from build123d import *

# Parameters (mm, degrees)
F1_W     = 65
F1_H     = 60
F1_R     = 2.5
F2_DEPTH = 1.5
F3_W     = 65
F3_H     = 1.5
F4_DEPTH = 25
F5_R     = 2
F6_DEPTH = 25
F7_R     = 2


with BuildPart() as f2:
    # F1 (on face) → F2 (new body)
    with BuildSketch(Plane.XZ):
        with Locations((32.5, -30)):
            Rectangle(F1_W, F1_H)
        with BuildLine():
            ThreePointArc((55, -45), (57.5, -47.5), (55, -50))
            ThreePointArc((55, -50), (34.847457, -41.652543), (26.5, -21.5))
            ThreePointArc((26.5, -21.5), (29, -19), (31.5, -21.5))
            ThreePointArc((31.5, -21.5), (38.382991, -38.117009), (55, -45))
        make_face(mode=Mode.SUBTRACT)
        with Locations((55, -21.5)):
            Circle(F1_R, mode=Mode.SUBTRACT)
    extrude(amount=F2_DEPTH)

    # F3 (on Front) → F4 (join)
    with BuildSketch(Plane.XZ):
        with Locations((32.5, -0.75)):
            Rectangle(F3_W, F3_H)
    extrude(amount=-F4_DEPTH)

    # F5 (on face) → F6 (cut)
    with BuildSketch(Plane.XY):
        with Locations((53, 12.5)):
            Circle(F5_R)
        with Locations((12, 12.5)):
            Circle(F5_R)
    extrude(amount=-F6_DEPTH, mode=Mode.SUBTRACT)

    # F7
    f7_edges = [f2.edges().sort_by_distance(p)[0] for p in [
        (65, -0.75, -60),
        (32.5, 0, -1.5),
        (32.5, -1.5, 0),
        (0, -0.75, -60),
        (0, 25, -0.75),
        (65, 25, -0.75),
    ]]
    fillet(f7_edges, radius=F7_R)


solid = f2.part
Geometry: final body of the model. Coordinates: model frame, mm. A direction names the side the tool comes from. Give positions to 0.01 mm unless a question says otherwise; leave off trailing zeros. Order: outer loops, then holes, each group sorted by start corner. A loop starts at its lowest first (then second) coordinate and runs counter-clockwise, first axis right, second up. Notation, with made-up numbers: (1, -0.5) - (9, -0.5) arc R15 cw to (9, 16.5) - close; hole circle Ø4 at (-15.75, 67). An arc over 180 degrees is marked (long way). Use CSV: the item, a comma, the result in double quotes.
1. Section query B-B (y = 13.5). Output: boundary loops of the cut face in (x, z).
Answers below:
outline,"(0, -1.5) - (10.27, -1.5) - (10.27, 0) - (0, 0) - close; (13.73, -1.5) - (51.27, -1.5) - (51.27, 0) - (13.73, 0) - close; (54.73, -1.5) - (65, -1.5) - (65, 0) - (54.73, 0) - close"
2. Section query C-C (z = -47.5). Output: boundary loops of the cut face in (x, y).
Answers below:
outline,"(0, -1.5) - (43.33, -1.5) - (43.33, 0) - (0, 0) - close; (57.5, -1.5) - (65, -1.5) - (65, 0) - (57.5, 0) - close"
3. Contact query for flat-ended pins moving along their axis: pin 1 (5 mm diameter, centred on x = 14, y = 22, fed in from -Z); pin 2 (3 mm diameter, centred on x = 51.5, y = 2.5, fed in from -Z). Output: stop coordinate, or through.
Answers below:
pin 1,"z = -1.5"
pin 2,"z = -1.77"
4. Mould query, pull axis Z, two halves, no side actions, for faces 1 (the face through (0.57, -0.76, -59.4)), 2 (the face through (35.1, -0.7, -41.9)), 3 (the face through (10.526, 13.852, -0.74)). Classes: +Z half, -Z half, draft (parallel to the pull), parting line (faces both ways), or undercut.
Answers below:
face 1,"-Z half"
face 2,"undercut"
face 3,"draft"
5. Access query for faces 4 (the face through (32, 0, -25)), 5 (the face through (0.57, 24.4, -0.74)), 6 (the face through (38.2, -0.74, -37.93)). Directions: +Z, -Z, +X, -X, +Y, -Y. A direction counts if a zero-diameter tool reaches every point of the face in a straight line with its end or side. Return the directions, or none.
Answers below:
face 4,"-Z, +X, -X, +Y"
face 5,"+Z, -Z, -X, +Y"
face 6,"+Y, -Y"
6. Material intervals for line 1 along Y through (x, z) = (32.5, -24); line 2 along Y through (x, z) = (53, -0.85), sorted ascending. Write a range as from..to.
Answers below:
line 1,"-1.5..0"
line 2,"-1.14..10.5, 14.5..25"
7. Section query A-A (z = -23). Output: boundary loops of the cut face in (x, y).
Answers below:
outline,"(0, -1.5) - (26.54, -1.5) - (26.54, 0) - (0, 0) - close; (31.55, -1.5) - (53, -1.5) - (53, 0) - (31.55, 0) - close; (57, -1.5) - (65, -1.5) - (65, 0) - (57, 0) - close"
8. Section query D-D (y = 6.25). Output: boundary loops of the cut face in (x, z), plus the area to 3 significant figures.
Answers below:
outline,"(0, -1.5) - (65, -1.5) - (65, 0) - (0, 0) - close"
area,"97.5 mm2"
